Verification items for this drawing (mm, ordinates from the low corner). Round coordinates to 2 decimals unless told otherwise and drop trailing zeros. Order: outer loops, then holes, each group sorted by start corner. A loop starts at its lowest first (then second) coordinate and runs counter-clockwise, first axis right, second up. Notation, with made-up numbers: (-10, 10) -> (24, 10) arc R21 cw to (24, 35) -> close; hole circle Ø3 at (79.5, 29.5). An arc over 180 degrees is marked (long way). Answer in a Markdown table with one row per item.
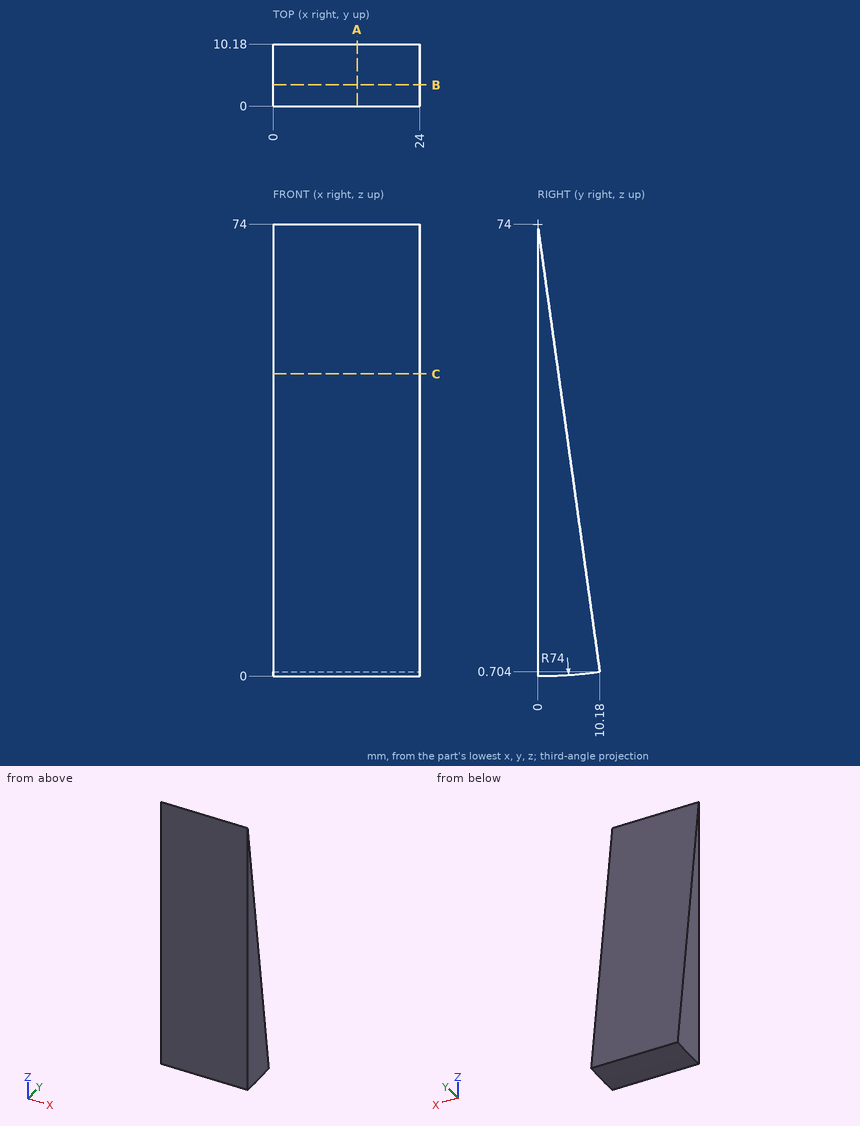
Item 1: Depth check by flat-ended pin: P1, Ø1, axis at x = 17, z = 30.5, coming from the +Y side; P2, Ø1.5, axis at y = 4.5, z = 58, coming from the -X side. Enter the tip coordinate at first touch or a pass-through.
Result sheet:
| item | result |
|---|---|
| P1 | stops at y = 6.11 |
| P2 | passes through |
Item 2: Cross-section at B-B (y = 3.5). Record the boundary of the cut face in (x, z), and give its area (3 significant figures).
Result sheet:
| item | result |
|---|---|
| outline | (0, 0.08) -> (24, 0.08) -> (24, 48.8) -> (0, 48.8) -> close |
| area | 1,170 mm^2 |
Item 3: Scan lines: line 1 (Y direction, x = 3, z = 39.5); line 2 (Y direction, x = 2, z = 11.5). Record each from-to range of solid material in increasing order. Write a range as [from, to].
Result sheet:
| item | result |
|---|---|
| line 1 | y = [0, 4.79] |
| line 2 | y = [0, 8.68] |
Item 4: Cross-section at A-A (x = 13.75). Record the boundary of the cut face in (y, z), and give its area (3 significant figures).
Result sheet:
| item | result |
|---|---|
| outline | (0, 0) arc R74 ccw to (10.18, 0.7) -> (0, 74) -> close |
| area | 378 mm^2 |
Item 5: Cross-section at C-C (z = 49.5). Record the boundary of the cut face in (x, y).
Result sheet:
| item | result |
|---|---|
| outline | (0, 0) -> (24, 0) -> (24, 3.4) -> (0, 3.4) -> close |
